Geometry check sheet. Reference: the model listing, model coordinates, mm. A direction names the side the tool comes from. Give positions to 0.01 mm unless a question says otherwise; leave off trailing zeros. Loops run counter-clockwise (first coordinate to the right, second up) from the corner with the lowest first, then second, coordinate; pieces in that order, holes last. Notation, with made-up numbers: (59.5, -13.75) -> (73.5, -13.75) arc R15 cw to (73.5, -5.75) -> close; hole circle Ø1 at (6.25, -27.75). An arc over 180 degrees is marked (long way). Write each question's results on one line, items separated by ' | '. Start each with the question number.
1) Sectioned sample at D-D on y = 3.5. Count the separate pieces of the cut face and the enclosed holes in it, then the cut area to 3 significant figures.
2) Depth check by flat-ended pin: pin 1 (1.9 mm diameter, centred on x = 137, y = 2, fed in from -Z); pin 2 (1.9 mm diameter, centred on x = 3.5, y = 2, fed in from +Z) (3 decimals); pin 3 (3 mm diameter, centred on y = 2, z = -2, fed in from -X). Enter the tip coordinate at first touch or a pass-through.
3) Draft check along Z on faces 5 (the face through (6.35, 3, -84)), 6 (the face through (3, 3, -53.975)), 7 (the face through (102, 3, -95.25)), 8 (the face through (13, 3, -6.35)). Enter one of: pulls with the +Z half, pulls with the -Z half, needs draft (parallel to the pull), parting line crosses it, or undercut.
4) Sectioned sample at C-C on z = -52. Record the cut outline in (x, y).
5) Sectioned sample at B-B on x = 116.65. Record the cut outline in (y, z).
6) Set-up check for faces 1 (the face through (184.15, 3, -48)), 2 (the face through (31.75, 3, -92)), 3 (the face through (171.45, 3, -3)), 4 (the face through (55.825, 3, -73)): record each of +Z, -Z, +X, -X, +Y, -Y from which the full face is reachable in a straight line by a thin tool's end or side.
7) Scan lines: line 1 (X direction, y = 0.5, z = -66); line 2 (Z direction, x = 52.65, y = 4.75); line 3 (Z direction, x = 91.5, y = 3.25). Record each from-to range of solid material in increasing order. Write a range as from..to.
8) Sectioned sample at A-A on z = -31.75. Record the cut outline in (x, y), then the cut area to 3 significant figures.
```python
from build123d import *

# Parameters (mm, degrees)
SKETCH1_W           = 431.8
SKETCH1_H           = 95.25
BOSS_EXTRUDE1_DEPTH = 6.35
SKETCH2_W           = 12.7
SKETCH2_H           = 6.35
CUT_EXTRUDE1_DEPTH  = 7.35
LPATTERN1_COUNT     = 17
LPATTERN1_PITCH     = 25.4
SKETCH3_W           = 6.35
SKETCH3_H           = 6.35
CUT_EXTRUDE2_DEPTH  = 7.35
SKETCH5_W           = 6.35
SKETCH5_H           = 12.7
CUT_EXTRUDE4_DEPTH  = 7.35
LPATTERN2_COUNT     = 2
LPATTERN2_PITCH     = 25.4
LPATTERN2_COL_COUNT = 2
LPATTERN2_COL_PITCH = 25.4
SKETCH6_W           = 114.3
SKETCH6_H           = 46.0375
CUT_EXTRUDE5_DEPTH  = 7.35
SKETCH7_R           = 1.75
CUT_EXTRUDE6_DEPTH  = 7.35
SKETCH8_W           = 6.35
SKETCH8_H           = 9.525
SKETCH8_H_2         = 12.7
CUT_EXTRUDE7_DEPTH  = 7.35
LPATTERN3_COUNT     = 2
LPATTERN3_PITCH     = 425.45
SKETCH9_W           = 241.3
SKETCH9_H           = 95.25
CUT_EXTRUDE8_DEPTH  = 7.35
SKETCH11_W          = 6.35
SKETCH11_H          = 6.35
BOSS_EXTRUDE2_DEPTH = 6.35
SKETCH12_W          = 57.65
SKETCH12_H          = 19.05
CUT_EXTRUDE10_DEPTH = 7.35
FILLET1_R           = 2.54
SKETCH13_R          = 12.7
CUT_EXTRUDE11_DEPTH = 7.35


with BuildPart() as part:
    # Sketch1 → Boss-Extrude1 (new body)
    with BuildSketch(Plane(origin=(0, 0, 0), x_dir=(1, 0, 0), z_dir=(0, 1, 0))):
        with Locations((215.9, 47.625)):
            Rectangle(SKETCH1_W, SKETCH1_H)
    extrude(amount=BOSS_EXTRUDE1_DEPTH)

    # Sketch2 → Cut-Extrude1 (cut, through all)
    with BuildSketch(Plane(origin=(0, 6.35, 0), x_dir=(1, 0, 0), z_dir=(0, 1, 0))):
        with Locations((12.7, 92.075)):
            Rectangle(SKETCH2_W, SKETCH2_H)
        with Locations((12.7, 3.175)):
            Rectangle(SKETCH2_W, SKETCH2_H)
    cut_extrude1 = extrude(amount=-CUT_EXTRUDE1_DEPTH, mode=Mode.SUBTRACT)

    # LPattern1: Cut-Extrude1 ×17
    with Locations(*[(i * LPATTERN1_PITCH, 0, 0) for i in range(1, LPATTERN1_COUNT)]):
        add(cut_extrude1, mode=Mode.SUBTRACT)

    # Sketch3 → Cut-Extrude2 (cut, through all)
    with BuildSketch(Plane(origin=(0, 6.35, 0), x_dir=(1, 0, 0), z_dir=(0, 1, 0))):
        with Locations((3.175, 92.075)):
            Rectangle(SKETCH3_W, SKETCH3_H)
        with Locations((3.175, 3.175)):
            Rectangle(SKETCH3_W, SKETCH3_H)
        with Locations((428.625, 92.075)):
            Rectangle(SKETCH3_W, SKETCH3_H)
        with Locations((428.625, 3.175)):
            Rectangle(SKETCH3_W, SKETCH3_H)
    extrude(amount=-CUT_EXTRUDE2_DEPTH, mode=Mode.SUBTRACT)

    # Sketch5 → Cut-Extrude4 (cut, through all)
    with BuildSketch(Plane(origin=(0, 6.35, 0), x_dir=(1, 0, 0), z_dir=(0, 1, 0))):
        with Locations((187.325, 47.625)):
            Rectangle(SKETCH5_W, SKETCH5_H)
        with Locations((307.975, 47.625)):
            Rectangle(SKETCH5_W, SKETCH5_H)
    cut_extrude4 = extrude(amount=-CUT_EXTRUDE4_DEPTH, mode=Mode.SUBTRACT)

    # LPattern2: Cut-Extrude4 ×2
    with Locations(*[(0, 0, -i * LPATTERN2_PITCH) for i in range(1, LPATTERN2_COUNT)]):
        add(cut_extrude4, mode=Mode.SUBTRACT)

    # LPattern2 col: Cut-Extrude4 ×2
    with Locations(*[(0, 0, i * LPATTERN2_COL_PITCH) for i in range(1, LPATTERN2_COL_COUNT)]):
        add(cut_extrude4, mode=Mode.SUBTRACT)

    # Sketch6 → Cut-Extrude5 (cut, through all)
    with BuildSketch(Plane(origin=(0, 6.35, 0), x_dir=(1, 0, 0), z_dir=(0, 1, 0))):
        with Locations((247.65, 47.625)):
            Rectangle(SKETCH6_W, SKETCH6_H)
    extrude(amount=-CUT_EXTRUDE5_DEPTH, mode=Mode.SUBTRACT)

    # Sketch7 → Cut-Extrude6 (cut, through all)
    with BuildSketch(Plane(origin=(0, 6.35, 0), x_dir=(1, 0, 0), z_dir=(0, 1, 0))):
        with Locations((52.65, 44.45)):
            Circle(SKETCH7_R)
        with Locations((116.65, 44.45)):
            Circle(SKETCH7_R)
        with Locations((315.15, 44.45)):
            Circle(SKETCH7_R)
        with Locations((379.15, 44.45)):
            Circle(SKETCH7_R)
    extrude(amount=-CUT_EXTRUDE6_DEPTH, mode=Mode.SUBTRACT)

    # Sketch8 → Cut-Extrude7 (cut, through all)
    with BuildSketch(Plane(origin=(0, 6.35, 0), x_dir=(1, 0, 0), z_dir=(0, 1, 0))):
        with Locations((3.175, 84.1375)):
            Rectangle(SKETCH8_W, SKETCH8_H)
        with Locations((3.175, 11.1125)):
            Rectangle(SKETCH8_W, SKETCH8_H)
        with Locations((3.175, 34.925)):
            Rectangle(SKETCH8_W, SKETCH8_H_2)
        with Locations((3.175, 60.325)):
            Rectangle(SKETCH8_W, SKETCH8_H_2)
    cut_extrude7 = extrude(amount=-CUT_EXTRUDE7_DEPTH, mode=Mode.SUBTRACT)

    # LPattern3: Cut-Extrude7 ×2
    with Locations(*[(i * LPATTERN3_PITCH, 0, 0) for i in range(1, LPATTERN3_COUNT)]):
        add(cut_extrude7, mode=Mode.SUBTRACT)

    # Sketch9 → Cut-Extrude8 (cut, through all)
    with BuildSketch(Plane(origin=(0, 6.35, 0), x_dir=(1, 0, 0), z_dir=(0, 1, 0))):
        with Locations((311.15, 47.625)):
            Rectangle(SKETCH9_W, SKETCH9_H)
    extrude(amount=-CUT_EXTRUDE8_DEPTH, mode=Mode.SUBTRACT)

    # Sketch11 → Boss-Extrude2 (add, through all)
    with BuildSketch(Plane(origin=(0, 6.35, 0), x_dir=(1, 0, 0), z_dir=(0, 1, 0))):
        with Locations((187.325, 92.075)):
            Rectangle(SKETCH11_W, SKETCH11_H)
    extrude(amount=-BOSS_EXTRUDE2_DEPTH)

    # Sketch12 → Cut-Extrude10 (cut, through all)
    with BuildSketch(Plane(origin=(0, 6.35, 0), x_dir=(1, 0, 0), z_dir=(0, 1, 0))):
        with Locations((84.65, 73.025)):
            Rectangle(SKETCH12_W, SKETCH12_H)
    extrude(amount=-CUT_EXTRUDE10_DEPTH, mode=Mode.SUBTRACT)

    # Fillet1
    fillet1_edges = [part.edges().sort_by_distance(p)[0] for p in [
        (55.825, 3.175, -63.5),
        (55.825, 3.175, -82.55),
        (113.475, 3.175, -82.55),
        (113.475, 3.175, -63.5),
    ]]
    fillet(fillet1_edges, radius=FILLET1_R)

    # Sketch13 → Cut-Extrude11 (cut, through all)
    with BuildSketch(Plane(origin=(0, 6.35, 0), x_dir=(1, 0, 0), z_dir=(0, 1, 0))):
        with Locations((158.75, 31.75)):
            Circle(SKETCH13_R)
    extrude(amount=-CUT_EXTRUDE11_DEPTH, mode=Mode.SUBTRACT)


solid = part.part
```
Result:
1) separate pieces: 1 | enclosed holes: 4 | area: 14,800 mm^2
2) pin 1: z = -88.9 | pin 2: z = -15.875 | pin 3: x = 19.05
3) face 5: needs draft | face 6: undercut | face 7: pulls with the -Z half | face 8: pulls with the +Z half
4) outline: (0, 0) -> (184.15, 0) -> (184.15, 6.35) -> (0, 6.35) -> close
5) outline: (0, -88.9) -> (6.35, -88.9) -> (6.35, -46.2) -> (0, -46.2) -> close; (0, -42.7) -> (6.35, -42.7) -> (6.35, -6.35) -> (0, -6.35) -> close
6) face 1: +X, +Y, -Y | face 2: -Z, +Y, -Y | face 3: +Z, +Y, -Y | face 4: +Y, -Y
7) line 1: 6.35..55.83, 113.47..190.5 | line 2: -95.25..-46.2, -42.7..0 | line 3: -88.9..-82.55, -63.5..-6.35
8) outline: (6.35, 0) -> (146.05, 0) -> (146.05, 6.35) -> (6.35, 6.35) -> close; (171.45, 0) -> (190.5, 0) -> (190.5, 6.35) -> (171.45, 6.35) -> close | area: 1,010 mm^2
